Build history of the part. All positions in model axes, mm. Round coordinates to 2 decimals unless told otherwise and drop trailing zeros. Write each loop counter-clockwise with the first axis right and the second up, starting at its lowest first coordinate (ties: lowest second). Pieces come first, ordered by that corner, then holes.
1) Saw through at B-B (z = 6.25). Write the cut outline in (x, y).
2) Flat gauge pins, fed straight in: pin 1 (5 mm diameter, centred on y = -12, z = 3.5, fed in from -X); pin 2 (5 mm diameter, centred on y = -34.5, z = 6.5, fed in from +X); pin 3 (1 mm diameter, centred on x = 5.5, z = 1.5, fed in from -Y). Where does each tip first touch, or does it go through?
3) Saw through at C-C (x = 3). Write the cut outline in (y, z), plus the area to 3 significant figures.
4) Saw through at D-D (y = -22.5). Write the cut outline in (x, z).
5) Saw through at A-A (x = 11.5). Write the cut outline in (y, z) (3 decimals).
6) Wall check: probe 1 along X at (y, z) = (-23, 5.75); probe 2 along Y at (x, z) = (20, 6); probe 3 along Y at (x, z) = (12, 10.5). Give the ranges that are in metal, low to high.
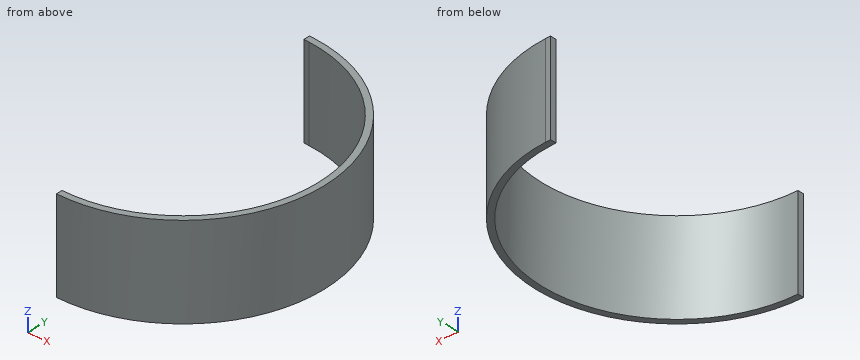
from build123d import *

# Parameters (mm, degrees)
SKETCH_1_R          = 1
EXTRUDE_1_DEPTH     = 15
EXTRUDE_2_DEPTH     = 15
CUT_EXTRUDE_1_DEPTH = 16


with BuildPart() as part:
    # ｽｹｯﾁ1 → ﾎﾞｽ - 押し出し1 (new body)
    with BuildSketch(Plane.XY):
        Circle(SKETCH_1_R)
    extrude(amount=EXTRUDE_1_DEPTH)

    # ｽｹｯﾁ2 → ﾎﾞｽ - 押し出し2 (add)
    with BuildSketch(Plane.XY.offset(15)):
        with BuildLine():
            Line((0, -44.5), (0, -45.5))
            ThreePointArc((0, -45.5), (23, -22.5), (0, 0.5))
            Line((0, 0.5), (0, -0.5))
            ThreePointArc((0, -0.5), (22, -22.5), (0, -44.5))
        make_face()
    extrude(amount=-EXTRUDE_2_DEPTH)

    # ｽｹｯﾁ6 → ｶｯﾄ - 押し出し1 (cut, through all)
    with BuildSketch(Plane.XY.offset(15)):
        with BuildLine():
            Line((0, 0.5), (0, -0.5))
            ThreePointArc((0, -0.5), (0.428174419, -0.504167061), (0.856186636, -0.516666667))
            Line((0.856186636, -0.516666667), (0.856186636, -1.684394884))
            Line((0.856186636, -1.684394884), (-3.351649942, -1.684394884))
            Line((-3.351649942, -1.684394884), (-3.351649942, 1.730475854))
            Line((-3.351649942, 1.730475854), (0.875436399, 1.730475854))
            Line((0.875436399, 1.730475854), (0.875436399, 0.483333333))
            ThreePointArc((0.875436399, 0.483333333), (0.437797518, 0.495832956), (0, 0.5))
        make_face()
    extrude(amount=-CUT_EXTRUDE_1_DEPTH, mode=Mode.SUBTRACT)


solid = part.part
Evaluation:
1. outline: (0, -45.5) arc R23 ccw to (0.88, 0.48) arc R23 ccw to (0, 0.5) - (0, -0.5) arc R22 cw to (0.86, -0.52) arc R22 cw to (0, -44.5) - close
2. pin 1: stops at x = 17.75
2. pin 2: stops at x = 20.95
2. pin 3: stops at y = -44.95
3. outline: (-45.3, 0) - (-44.29, 0) - (-44.29, 15) - (-45.3, 15) - close; (-0.71, 0) - (0.3, 0) - (0.3, 15) - (-0.71, 15) - close
3. area: 30.3 mm2
4. outline: (22, 0) - (23, 0) - (23, 15) - (22, 15) - close
5. outline: (-42.419, 0) - (-41.255, 0) - (-41.255, 15) - (-42.419, 15) - close; (-3.745, 0) - (-2.581, 0) - (-2.581, 15) - (-3.745, 15) - close
6. probe 1: x = 21.99 to 22.99
6. probe 2: y = -33.86 to -31.67, -13.33 to -11.14
6. probe 3: y = -42.12 to -40.94, -4.06 to -2.88
